Could you check a few things on this model? Use its own coordinates, in mm. A direction names the side the tool comes from. Give positions to 0.01 mm unless a question says otherwise; leave off trailing zeros. Order: outer loops, then holes, each group sorted by start corner. A loop starts at its lowest first (then second) coordinate and runs counter-clockwise, first axis right, second up.
(1) Imagine slicing it at C-C, the plane x = 8.5. Write out the boundary of the cut face in (y, z), then the cut area to 3 significant figures.
(2) Imagine slicing it at A-A, the plane y = 8. Write out the boundary of the cut face in (x, z), then the cut area to 3 significant figures.
(3) Imagine slicing it at D-D, the plane y = 18.5. Write out the boundary of the cut face in (x, z), then the cut area to 3 significant figures.
(4) If I drill on probe 1 along Z at (x, y) = (38.5, 32.5); probe 2 along X at (y, z) = (16, 12); probe 3 along Y at (x, z) = (4.5, 20.5), over which ranges is the centre line in solid material (lowest first)?
(5) Will these pins go through, and if not, where does the flat tip stop? pin 1 (5 mm diameter, centred on y = 6.5, z = 8, fed in from +X); pin 2 (2 mm diameter, centred on x = 29, y = 14.5, fed in from +Z); pin 3 (0.6 mm diameter, centred on x = 60, y = 1.5, fed in from +Z).
(6) If we mould it in two halves opening along Z, with no side actions, what happens to faces 1 (the flat face through (52, 29, 30)), 2 (the flat face through (64, 24, 11)), 3 (the flat face through (60, 1, 19))? For each: released by +Z, released by -Z, zero draft, split by the parting line, or undercut.
(7) On a 3-axis mill with a long thin cutter (end or side, diameter ignored), from which of +Z, -Z, +X, -X, +Y, -Y can I reach the whole of each face in a straight line? I mean faces 4 (the flat face through (58, 1, 12)), 5 (the flat face through (32, 42, 11)), 6 (the flat face through (60, 38, 25)). Say none if no direction works.
(8) Imagine slicing it at B-B, the plane z = 8. Write out the boundary of the cut face in (x, y).
from build123d import *

# Parameters (mm, degrees)
SKETCH1_W           = 64
SKETCH1_H           = 42
BOSS_EXTRUDE1_DEPTH = 25
FILLET2_R           = 5
FILLET4_R           = 3
BOSS_EXTRUDE3_START = -3
SKETCH2_R           = 11.5
BOSS_EXTRUDE3_DEPTH = 8
SKETCH3_W           = 15
SKETCH3_H           = 21
CUT_EXTRUDE1_DEPTH  = 1
SKETCH4_W           = 15
SKETCH4_H           = 2
CUT_EXTRUDE2_DEPTH  = 5


with BuildPart() as part:
    # Sketch1 → Boss-Extrude1 (new body)
    with BuildSketch(Plane.XY):
        with Locations((32, 21)):
            Rectangle(SKETCH1_W, SKETCH1_H)
    extrude(amount=BOSS_EXTRUDE1_DEPTH)

    # Fillet2
    fillet2_edges = [part.edges().sort_by_distance(p)[0] for p in [
        (0, 42, 12.5),
        (64, 42, 12.5),
        (64, 0, 12.5),
        (0, 0, 12.5),
    ]]
    fillet(fillet2_edges, radius=FILLET2_R)

    # Fillet4
    fillet4_edges = [part.edges().sort_by_distance(p)[0] for p in [
        (64, 21, 25),
        (32, 0, 25),
        (0, 21, 25),
        (32, 42, 25),
        (62.535533906, 40.535533906, 25),
        (1.464466094, 40.535533906, 25),
        (1.464466094, 1.464466094, 25),
        (62.535533906, 1.464466094, 25),
    ]]
    fillet(fillet4_edges, radius=FILLET4_R)

    # Sketch2 → Boss-Extrude3 (add)
    with BuildSketch(Plane.XY.offset(25).offset(BOSS_EXTRUDE3_START)):
        with Locations((52.5, 29)):
            Circle(SKETCH2_R)
    extrude(amount=BOSS_EXTRUDE3_DEPTH)

    # Sketch3 → Cut-Extrude1 (cut)
    with BuildSketch(Plane(origin=(64, 0, 0), x_dir=(0, 0, -1), z_dir=(1, 0, 0))):
        with Locations((-11.5, 10.5)):
            Rectangle(SKETCH3_W, SKETCH3_H)
    extrude(amount=-CUT_EXTRUDE1_DEPTH, mode=Mode.SUBTRACT)

    # Sketch4 → Cut-Extrude2 (cut)
    with BuildSketch(Plane(origin=(63, 0, 0), x_dir=(0, 0, -1), z_dir=(1, 0, 0))):
        with Locations((-11.5, 1)):
            Rectangle(SKETCH4_W, SKETCH4_H)
    extrude(amount=-CUT_EXTRUDE2_DEPTH, mode=Mode.SUBTRACT)


solid = part.part
Answer block:
1. outline: (0, 0) - (42, 0) - (42, 22) arc R3 ccw to (39, 25) - (3, 25) arc R3 ccw to (0, 22) - close
1. area: 1,050 mm2
2. outline: (0, 0) - (64, 0) - (64, 4) - (63, 4) - (63, 19) - (64, 19) - (64, 22) arc R3 ccw to (61, 25) - (3, 25) arc R3 ccw to (0, 22) - close
2. area: 1,580 mm2
3. outline: (0, 0) - (64, 0) - (64, 4) - (63, 4) - (63, 19) - (64, 19) - (64, 22) arc R3 ccw to (61, 25) - (57.19, 25) - (57.19, 30) - (47.81, 30) - (47.81, 25) - (3, 25) arc R3 ccw to (0, 22) - close
3. area: 1,630 mm2
4. probe 1: z = 0 to 25
4. probe 2: x = 0 to 63
4. probe 3: y = 0.03 to 41.97
5. pin 1: stops at x = 63
5. pin 2: stops at z = 25
5. pin 3: stops at z = 24.68
6. face 1: released by +Z
6. face 2: zero draft
6. face 3: undercut
7. face 4: +X, -Y
7. face 5: +Z, -Z, +X, -X, +Y
7. face 6: +Z, +X, +Y
8. outline: (0, 5) arc R5 ccw to (5, 0) - (58, 0) - (58, 2) - (63, 2) - (63, 21) - (64, 21) - (64, 37) arc R5 ccw to (59, 42) - (5, 42) arc R5 ccw to (0, 37) - close
